The listing builds one solid part. Answer for the finished solid, in the listing's coordinates (mm). A direction names the side the tool comes from. Coordinates: 2 decimals unless noted, no trailing zeros. Loops run counter-clockwise (first coordinate to the right, second up) from the corner with the lowest first, then second, coordinate; pieces in that order, holes last. Notation, with made-up numbers: (45, -27.75) - (57, -27.75) arc R18 ccw to (57, -19.75) - close; hole circle Ø2 at (13, -28.5). An arc over 180 degrees is marked (long way). One line per question, with ' | ' between items.
from build123d import *

# Parameters (mm, degrees)
F0_R     = 25.410924
F1_DEPTH = 268.732
F2_R     = 21.364523
F3_DEPTH = 1270
F5_DEPTH = 142240


with BuildPart() as f1:
    # F0 (on Top) → F1 (new body)
    with BuildSketch(Plane.XY):
        Circle(F0_R)
    extrude(amount=F1_DEPTH)

    # F2 (on face) → F3 (cut)
    with BuildSketch(Plane.XY.offset(268.732)):
        Circle(F2_R)
    extrude(amount=-F3_DEPTH, mode=Mode.SUBTRACT)

    # F4 (on face) → F5 (cut)
    with BuildSketch(Plane.XY.offset(268.732)):
        Polygon((0, 32.184474), (-14.504612, 15.68627), (14.643387, 15.68627), align=None)
    extrude(amount=-F5_DEPTH, mode=Mode.SUBTRACT)


solid = f1.part
Item 1: The mould has two halves that part along X. Classify faces 1 (the face through (-8, -21, 268.732)), 2 (the face through (-1.07, -25.39, 132.48)), 3 (the face through (10.799, 20.017, 136.247)): pulls with the +X half, pulls with the -X half, needs draft (parallel to the pull), parting line crosses it, or undercut.
Taken from the geometry:
face 1: needs draft | face 2: parting line crosses it | face 3: undercut
Item 2: Find section B-B, the plane z = 227. Write down the section's boundary in (x, y), plus the area to 3 significant figures.
Taken from the geometry:
outline: (-14.5, 15.69) - (-6.76, 24.5) arc R25.41 ccw (long way) to (6.85, 24.47) - (14.64, 15.69) - (14.5, 15.69) arc R21.36 cw (long way) to start | area: 511 mm2
Item 3: Which of the six approach directions +Z, -Z, +X, -X, +Y, -Y give full straight-line access (tool end or side, diameter ignored) to faces 4 (the face through (-10.58, 20.15, 136.25)), 5 (the face through (-8, -21, 0))?
Taken from the geometry:
face 4: +Z, -Z | face 5: -Z, +X, -X, +Y, -Y
Item 4: Find the intervals of material crossed by line 1 (X direction, y = 0, z = 161.5); line 2 (Y direction, x = 0, z = 55); line 3 (Y direction, x = -7, z = 228.5), in increasing order. Write a range as [from, to].
Taken from the geometry:
line 1: x = [-25.41, -21.36], [21.36, 25.41] | line 2: y = [-25.41, -21.36] | line 3: y = [-24.43, -20.19], [24.22, 24.43]
Item 5: Find section C-C, the plane x = 0. Write down the section's boundary in (y, z).
Taken from the geometry:
outline: (-25.41, 0) - (-21.36, 0) - (-21.36, 268.73) - (-25.41, 268.73) - close
Item 6: Each of these flat-tipped pins is pushed along its axis until it touches: pin 1 Ø3 at (x, z) = (-10.5, 71) entering from -Y; pin 2 Ø1 at (x, z) = (3, 191.5) entering from +Y; pin 3 Ø12 at (x, z) = (15, 36.5) entering from +Y; pin 4 Ø5 at (x, y) = (19.5, 19) entering from -Z. Where does it stop, or does it pass through?
Taken from the geometry:
pin 1: stops at y = -23.76 | pin 2: stops at y = -21.08 | pin 3: stops at y = 23.76 | pin 4: stops at z = 0
Item 7: Find section A-A, the plane y = 0. Write down the section's boundary in (x, z).
Taken from the geometry:
outline: (-25.41, 0) - (-21.36, 0) - (-21.36, 268.73) - (-25.41, 268.73) - close; (21.36, 0) - (25.41, 0) - (25.41, 268.73) - (21.36, 268.73) - close
